Can you work these out from the model? Positions are in its coordinate system, mm. A direction names the side the tool comes from. Give positions to 0.01 mm unless a question says otherwise; leave off trailing zeros. Write each loop counter-clockwise with the first axis right and the second up, starting at its lowest first coordinate (ties: lowest second). Pieces come first, ordered by that corner, then holes.
from build123d import *

# Parameters (mm, degrees)
SKETCH1_R                      = 35.75
SKETCH1_R_2                    = 1.7
BOSS_EXTRUDE1_DEPTH            = 10.8
CUT_EXTRUDE1_START             = -7.7
SKETCH2_R                      = 3
SKETCH2_R_2                    = 1.7
CUT_EXTRUDE1_DEPTH             = 7.7
SKETCH3_W                      = 6
SKETCH3_H                      = 10
CUT_EXTRUDE2_DEPTH             = 52.698791088
CUT_EXTRUDE3_DEPTH             = 52.698791088
CUT_EXTRUDE3_DIRECTION_2_REACH = 53.699
BOSS_EXTRUDE2_DEPTH            = 7.7
CUT_EXTRUDE4_DEPTH             = 66.040487391
CUT_EXTRUDE4_DEPTH_BACK        = 66.040487391
SKETCH6_W                      = 4.8
SKETCH6_H                      = 17.274998913
CUT_EXTRUDE5_DEPTH             = 66.040487391
CUT_EXTRUDE5_DEPTH_BACK        = 66.040487391
SKETCH8_W                      = 6
SKETCH8_H                      = 23.025515334
CUT_EXTRUDE6_DEPTH             = 10


with BuildPart() as part:
    # Sketch1 → Boss-Extrude1 (new body)
    with BuildSketch(Plane.XY):
        with Locations(Location((0, 0, 0), (0, 0, 180))):
            Circle(SKETCH1_R)
        with Locations(Location((0, 31, 0), (0, 0, 180))):
            Circle(SKETCH1_R_2, mode=Mode.SUBTRACT)
        with Locations(Location((31, 0, 0), (0, 0, 180))):
            Circle(SKETCH1_R_2, mode=Mode.SUBTRACT)
        with Locations(Location((0, -31, 0), (0, 0, 180))):
            Circle(SKETCH1_R_2, mode=Mode.SUBTRACT)
        with Locations(Location((-31, 0, 0), (0, 0, 180))):
            Circle(SKETCH1_R_2, mode=Mode.SUBTRACT)
    extrude(amount=BOSS_EXTRUDE1_DEPTH)

    # Sketch2 → Cut-Extrude1 (cut)
    # profile 1 of 4: a face of its own
    with BuildSketch(Plane.XY.offset(10.8).offset(CUT_EXTRUDE1_START)):
        with Locations((-31, 0)):
            Circle(SKETCH2_R)
        with Locations(Location((-31, 0, 0), (0, 0, 180))):
            Circle(SKETCH2_R_2, mode=Mode.SUBTRACT)
    # profile 2 of 4: a face of its own
    with BuildSketch(Plane.XY.offset(10.8).offset(CUT_EXTRUDE1_START)):
        with Locations((31, 0)):
            Circle(SKETCH2_R)
        with Locations(Location((31, 0, 0), (0, 0, 180))):
            Circle(SKETCH2_R_2, mode=Mode.SUBTRACT)
    # profile 3 of 4: a face of its own
    with BuildSketch(Plane.XY.offset(10.8).offset(CUT_EXTRUDE1_START)):
        with Locations((0, -31)):
            Circle(SKETCH2_R)
        with Locations(Location((0, -31, 0), (0, 0, 180))):
            Circle(SKETCH2_R_2, mode=Mode.SUBTRACT)
    # profile 4 of 4: a face of its own
    with BuildSketch(Plane.XY.offset(10.8).offset(CUT_EXTRUDE1_START)):
        with Locations((0, 31)):
            Circle(SKETCH2_R)
    extrude(amount=CUT_EXTRUDE1_DEPTH, mode=Mode.SUBTRACT)

    # Sketch3 → Cut-Extrude2 (cut, through all)
    with BuildSketch(Plane.XY.offset(10.8)):
        with Locations((-20.5, 17)):
            Rectangle(SKETCH3_W, SKETCH3_H)
    extrude(amount=-CUT_EXTRUDE2_DEPTH, mode=Mode.SUBTRACT)

    # Sketch4 → Cut-Extrude3 (cut)
    with BuildSketch(Plane(origin=(0, 0, 0), x_dir=(1, 0, 0), z_dir=(0, 1, 0))):
        Polygon((35.75, -6), (17.3, -6), (23.06, -10.8), (35.75, -10.8), align=None)
        Polygon((23.06, -10.8), (22.947590013, -10.8), (17.187590013, -6), (17.3, -6), align=None)
        Polygon((-23.26, -10.8), (-17.5, -6), (-35.75, -6), (-35.75, -10.8), align=None)
        Polygon((-23.06, -10.8), (-17.3, -6), (-17.5, -6), (-23.26, -10.8), align=None)
        Polygon((-17.3, -6.093674989), (-17.3, -6), (-23.06, -10.8), (-22.947590013, -10.8), align=None)
    extrude(amount=-CUT_EXTRUDE3_DEPTH, mode=Mode.SUBTRACT)

    # Cut-Extrude3 direction 2: up to this face of the body (flat: up to its plane)
    cut_extrude3_direction_2_end = Plane(part.part.faces().sort_by_distance((-20.5, 22, 5.4))[0])
    # Sketch4 → Cut-Extrude3 direction 2 (cut, up to the picked face)
    with BuildSketch(Plane(origin=(0, 0, 0), x_dir=(1, 0, 0), z_dir=(0, 1, 0)), mode=Mode.PRIVATE) as cut_extrude3_direction_2_sk1:
        Polygon((35.75, -6), (17.3, -6), (23.06, -10.8), (35.75, -10.8), align=None)
    cut_extrude3_direction_2_tool1 = split(extrude(cut_extrude3_direction_2_sk1.sketch, amount=CUT_EXTRUDE3_DIRECTION_2_REACH, mode=Mode.PRIVATE), bisect_by=cut_extrude3_direction_2_end, keep=Keep.BOTH, mode=Mode.PRIVATE)
    # Sketch4 → Cut-Extrude3 direction 2 (cut, up to the picked face)
    with BuildSketch(Plane(origin=(0, 0, 0), x_dir=(1, 0, 0), z_dir=(0, 1, 0)), mode=Mode.PRIVATE) as cut_extrude3_direction_2_sk2:
        Polygon((23.06, -10.8), (22.947590013, -10.8), (17.187590013, -6), (17.3, -6), align=None)
    cut_extrude3_direction_2_tool2 = split(extrude(cut_extrude3_direction_2_sk2.sketch, amount=CUT_EXTRUDE3_DIRECTION_2_REACH, mode=Mode.PRIVATE), bisect_by=cut_extrude3_direction_2_end, keep=Keep.BOTH, mode=Mode.PRIVATE)
    # Sketch4 → Cut-Extrude3 direction 2 (cut, up to the picked face)
    with BuildSketch(Plane(origin=(0, 0, 0), x_dir=(1, 0, 0), z_dir=(0, 1, 0)), mode=Mode.PRIVATE) as cut_extrude3_direction_2_sk3:
        Polygon((-23.26, -10.8), (-17.5, -6), (-35.75, -6), (-35.75, -10.8), align=None)
    cut_extrude3_direction_2_tool3 = split(extrude(cut_extrude3_direction_2_sk3.sketch, amount=CUT_EXTRUDE3_DIRECTION_2_REACH, mode=Mode.PRIVATE), bisect_by=cut_extrude3_direction_2_end, keep=Keep.BOTH, mode=Mode.PRIVATE)
    # Sketch4 → Cut-Extrude3 direction 2 (cut, up to the picked face)
    with BuildSketch(Plane(origin=(0, 0, 0), x_dir=(1, 0, 0), z_dir=(0, 1, 0)), mode=Mode.PRIVATE) as cut_extrude3_direction_2_sk4:
        Polygon((-23.06, -10.8), (-17.3, -6), (-17.5, -6), (-23.26, -10.8), align=None)
    cut_extrude3_direction_2_tool4 = split(extrude(cut_extrude3_direction_2_sk4.sketch, amount=CUT_EXTRUDE3_DIRECTION_2_REACH, mode=Mode.PRIVATE), bisect_by=cut_extrude3_direction_2_end, keep=Keep.BOTH, mode=Mode.PRIVATE)
    # Sketch4 → Cut-Extrude3 direction 2 (cut, up to the picked face)
    with BuildSketch(Plane(origin=(0, 0, 0), x_dir=(1, 0, 0), z_dir=(0, 1, 0)), mode=Mode.PRIVATE) as cut_extrude3_direction_2_sk5:
        Polygon((-17.3, -6.093674989), (-17.3, -6), (-23.06, -10.8), (-22.947590013, -10.8), align=None)
    cut_extrude3_direction_2_tool5 = split(extrude(cut_extrude3_direction_2_sk5.sketch, amount=CUT_EXTRUDE3_DIRECTION_2_REACH, mode=Mode.PRIVATE), bisect_by=cut_extrude3_direction_2_end, keep=Keep.BOTH, mode=Mode.PRIVATE)
    add(cut_extrude3_direction_2_tool1.solids().sort_by(Axis((27.876214, 0, 8.252023), (0, 1, 0)))[0], mode=Mode.SUBTRACT)
    add(cut_extrude3_direction_2_tool2.solids().sort_by(Axis((20.123795, 0, 8.4), (0, 1, 0)))[0], mode=Mode.SUBTRACT)
    add(cut_extrude3_direction_2_tool3.solids().sort_by(Axis((-27.975059, 0, 8.250098), (0, 1, 0)))[0], mode=Mode.SUBTRACT)
    add(cut_extrude3_direction_2_tool4.solids().sort_by(Axis((-20.28, 0, 8.4), (0, 1, 0)))[0], mode=Mode.SUBTRACT)
    add(cut_extrude3_direction_2_tool5.solids().sort_by(Axis((-20.15199, 0, 8.423342), (0, 1, 0)))[0], mode=Mode.SUBTRACT)

    # Sketch5 → Boss-Extrude2 (add)
    with BuildSketch(Plane.ZY.offset(17.5)):
        Polygon((6.260341656, 22), (6.166666667, 22), (6, 22), (6, 12), (6.260341656, 12), align=None)
    extrude(amount=-BOSS_EXTRUDE2_DEPTH)

    # Sketch6 → Cut-Extrude4 (cut, two sides: drawn at the far end of the back side and taken through both)
    with BuildSketch(Plane.ZY.offset(17.5).offset(-CUT_EXTRUDE4_DEPTH_BACK)):
        with Locations((8.4, 30.637499457)):
            Rectangle(SKETCH6_W, SKETCH6_H)
    extrude(amount=CUT_EXTRUDE4_DEPTH + CUT_EXTRUDE4_DEPTH_BACK, mode=Mode.SUBTRACT)

    # Sketch7 → Cut-Extrude5 (cut, two sides: drawn at the far end of the back side and taken through both)
    with BuildSketch(Plane.ZY.offset(17.5).offset(-CUT_EXTRUDE5_DEPTH_BACK)):
        Polygon((6, -3), (6, 0), (6, 3), (10.8, 3), (10.8, -3), align=None)
    extrude(amount=CUT_EXTRUDE5_DEPTH + CUT_EXTRUDE5_DEPTH_BACK, mode=Mode.SUBTRACT)

    # Sketch8 → Cut-Extrude6 (cut)
    with BuildSketch(Plane(origin=(0, 0, 0), x_dir=(-1, 0, 0), z_dir=(0, 0, -1))):
        with Locations((20.5, 23.512757667)):
            Rectangle(SKETCH8_W, SKETCH8_H)
    extrude(amount=-CUT_EXTRUDE6_DEPTH, mode=Mode.SUBTRACT)


solid = part.part
(1) Will these pins go through, and if not, where does the flat tip stop? P1, Ø6, axis at y = 4.5, z = 5, coming from the -X side; P2, Ø1.8, axis at y = 20.5, z = 3, coming from the +X side; P3, Ø3.5, axis at x = 0, y = -31, coming from the +Z side; P4, Ø4.5, axis at x = 31, y = 0, coming from the -Z side.
Returned:
P1: stops at x = -35.72
P2: stops at x = 29.9
P3: stops at z = 3.1
P4: stops at z = 0
(2) Imagine slicing it at C-C, the plane z = 9.75. Write out the boundary of the cut face in (x, y).
Returned:
outline: (-21.69, -28.42) arc R35.75 ccw to (21.69, -28.42) - (21.69, -3) - (-21.69, -3) - close; (-21.69, 3) - (21.69, 3) - (21.69, 22) - (-17.5, 22) - (-17.5, 12) - (-21.69, 12) - close; hole circle Ø6 at (0, -31)
(3) Imagine slicing it at D-D, the plane z = 4. Write out the boundary of the cut face in (x, y).
Returned:
outline: (-23.5, 12) - (-23.5, 26.94) arc R35.75 ccw (long way) to (-17.5, 31.17) - (-17.5, 12) - close; hole circle Ø6 at (-31, 0); hole circle Ø6 at (0, -31); hole circle Ø6 at (0, 31); hole circle Ø6 at (31, 0)
(4) Imagine slicing it at B-B, the plane x = 0. Write out the boundary of the cut face in (y, z), plus the area to 3 significant figures.
Returned:
outline: (-35.75, 0) - (-32.7, 0) - (-32.7, 3.1) - (-34, 3.1) - (-34, 10.8) - (-35.75, 10.8) - close; (-29.3, 0) - (29.3, 0) - (29.3, 3.1) - (28, 3.1) - (28, 6) - (22, 6) - (22, 10.8) - (3, 10.8) - (3, 6) - (-3, 6) - (-3, 10.8) - (-28, 10.8) - (-28, 3.1) - (-29.3, 3.1) - close; (32.7, 0) - (35.75, 0) - (35.75, 6) - (34, 6) - (34, 3.1) - (32.7, 3.1) - close
area: 593 mm2
(5) For faces 5 (the face through (-23.5, 19, 3)), 6 (the face through (0.37, -29.34, 1.53)), 7 (the face through (-29, 0, 3.1)), which set-ups out of +Z, -Z, +X, -X, +Y, -Y let a thin tool reach every point of the face, with its end or its side?
Returned:
face 5: +Z, -Z, +Y
face 6: +Z, -Z
face 7: +Z
(6) If I drill on L1, parallel to Y at x = 0, z = 5.25; L2, parallel to Z at x = 26, y = -8, over which ranges is the centre line in solid material (lowest first)?
Returned:
L1: y = -35.75 to -34, -28 to 28, 34 to 35.75
L2: z = 0 to 6
(7) If we mould it in two halves opening along Y, with no side actions, what happens to faces 1 (the face through (28, 0, 5)), 2 (the face through (-19, 12, 10)), 3 (the face through (0, -3, 8)), 4 (the face through (20.108, 12.633, 8.434))? For each: +Y half, -Y half, draft (parallel to the pull), parting line (faces both ways), or undercut.
Returned:
face 1: undercut
face 2: +Y half
face 3: undercut
face 4: draft
(8) Imagine slicing it at A-A, the plane y = 0. Write out the boundary of the cut face in (x, z), plus the area to 3 significant figures.
Returned:
outline: (-35.75, 0) - (-32.7, 0) - (-32.7, 3.1) - (-34, 3.1) - (-34, 6) - (-35.75, 6) - close; (-29.3, 0) - (29.3, 0) - (29.3, 3.1) - (28, 3.1) - (28, 6) - (-28, 6) - (-28, 3.1) - (-29.3, 3.1) - close; (32.7, 0) - (35.75, 0) - (35.75, 6) - (34, 6) - (34, 3.1) - (32.7, 3.1) - close
area: 373 mm2
